Part model, mm, in its own coordinate system. Face numbers are marked on the shaded views. A direction names the side the tool comes from. Coordinates: 2 decimals unless noted, no trailing zeros. Loops run counter-clockwise (first coordinate to the right, second up) from the corner with the lowest first, then second, coordinate; pieces in that order, holes last. Notation, with made-up numbers: (40.25, 45) - (96.25, 45) arc R22 cw to (96.25, 62) - close; hole circle Ø6 at (46.5, 35). An arc over 180 degrees is marked (long way). Use a Markdown table: item, result. Add a question column.
1) Probe probe 1 along Y at (x, z) = (86.5, 50.5); probe 2 along X at (y, z) = (-6.5, 7.5) (3 decimals); probe 3 along Z at (x, y) = (-3, 45.5) (3 decimals). List the from-to ranges inside material, lowest first. Write a range as [from, to].
2) Band-saw the part on B-B (y = 29). Give the cut face in (x, z) (3 decimals), plus the area to 3 significant figures.
3) Drop flat-ended pins along their axis: P1, Ø3, axis at y = 6.5, z = 24, coming from the +X side (3 decimals); P2, Ø6, axis at y = -22.5, z = 30.5, coming from the +X side; P3, Ø16, axis at x = 22.5, z = 40, coming from the +Y side. Give the stop position or say it passes through.
4) Band-saw the part on A-A (x = 87.5). Give the cut face in (y, z) (3 decimals), plus the area to 3 significant figures.
5) Tool access for the marked faces 1, 2, 3 and 4: list every direction of +Z, -Z, +X, -X, +Y, -Y with a clear straight run to the whole face (end or side of a thin tool).
6) Pull direction Y, two halves, no side cores. Call the marked faces 5, 6, 7 and 8: +Y half, -Y half, draft (parallel to the pull), parting line (faces both ways), or undercut.
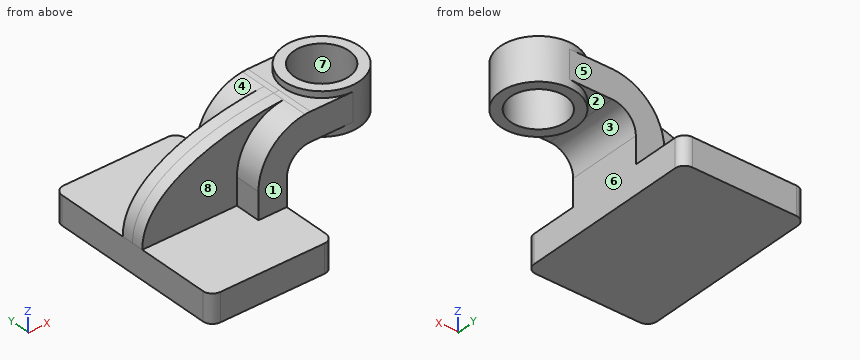
from build123d import *

# Parameters (mm, degrees)
F1_DEPTH = 63.5
F0_W     = 25.4
F0_H     = 19.05
F2_DEPTH = 25.4
F3_DEPTH = 7.9375
F5_R     = 6.35
F6_R     = 18.4889693292
F7_DEPTH = 100.96774064


with BuildPart() as f1:
    # F0 (on Front) → F1 (new body, symmetric)
    with BuildSketch(Plane.XZ):
        Polygon((41.275, -9.525), (41.275, 9.525), (22.225, 9.525), (-41.275, 9.525), (-41.275, -9.525), align=None)
    extrude(amount=F1_DEPTH, both=True)

    # F0 (on Front) → F2 (join, symmetric)
    with BuildSketch(Plane.XZ):
        with BuildLine():
            Line((22.225, 9.525), (41.275, 9.525))
            Line((41.275, 9.525), (41.275, 27.5082))
            ThreePointArc((41.275, 27.5082), (45.9246798487, 38.7335201513), (57.15, 43.3832))
            Line((57.15, 43.3832), (60.325, 43.3832))
            Line((60.325, 43.3832), (60.325, 62.4332))
            Line((60.325, 62.4332), (57.15, 62.4332))
            add(Edge.make_bspline(
                [(53.5324999081, 62.2453460843), (54.7490836223, 62.3182036116), (55.9554653988, 62.3807456949), (57.15, 62.4332)],
                knots=[108.5679461474, 108.5679461474, 108.5679461474, 108.5679461474, 111.7441642872, 111.7441642872, 111.7441642872, 111.7441642872], degree=3))
            ThreePointArc((53.5324999081, 62.2453460843), (31.2068234818, 50.8899710438), (22.225, 27.5082))
            Line((22.225, 27.5082), (22.225, 9.525))
        make_face()
        with Locations((73.025, 52.9082)):
            Rectangle(F0_W, F0_H)
    extrude(amount=F2_DEPTH, both=True)

    # F0 (on Front) → F3 (join, symmetric)
    with BuildSketch(Plane.XZ):
        with BuildLine():
            Line((-41.275, 9.525), (22.225, 9.525))
            Line((22.225, 9.525), (22.225, 27.5082))
            ThreePointArc((22.225, 27.5082), (31.2068234818, 50.8899710438), (53.5324999081, 62.2453460843))
            add(Edge.make_bspline(
                [(-41.275, 9.525), (-41.5565460879, 45.2122684176), (11.9478261389, 59.7549654652), (53.5324999081, 62.2453460843)],
                knots=[0, 0, 0, 0, 108.5679461474, 108.5679461474, 108.5679461474, 108.5679461474], degree=3))
        make_face()
    extrude(amount=F3_DEPTH, both=True)

    # F0 (on Front) → F4 (revolve)
    with BuildSketch(Plane.XZ):
        Polygon((85.725, 62.4332), (85.725, 43.3832), (85.725, 38.1), (111.125, 38.1), (111.125, 66.675), (85.725, 66.675), align=None)
    revolve(axis=Axis((85.725, 0, 52.3875), (0, 0, 1)))

    # F5
    f5_edges = [f1.edges().sort_by_distance(p)[0] for p in [
        (41.275, -63.5, 0),
        (-41.275, -63.5, 0),
        (-41.275, 63.5, 0),
        (41.275, 63.5, 0),
    ]]
    fillet(f5_edges, radius=F5_R)

    # F6 (on face) → F7 (cut)
    with BuildSketch(Plane.XY.offset(66.675)):
        with Locations((85.725, 0)):
            Circle(F6_R)
    extrude(amount=-F7_DEPTH, mode=Mode.SUBTRACT)


solid = f1.part
Answer block:
| question | item | result |
|---|---|---|
| 1 | probe 1 | [-25.39, -18.47], [18.47, 25.39] |
| 1 | probe 2 | [-41.275, 41.275] |
| 1 | probe 3 | [-9.525, 9.525] |
| 2 | outline | (-41.275, -9.525) - (41.275, -9.525) - (41.275, 9.525) - (-41.275, 9.525) - close |
| 2 | area | 1,570 mm2 |
| 3 | P1 | x = 41.275 |
| 3 | P2 | x = 42.45 |
| 3 | P3 | y = 25.4 |
| 4 | outline | (-25.338, 38.1) - (-18.404, 38.1) - (-18.404, 66.675) - (-25.338, 66.675) - close; (18.404, 38.1) - (25.338, 38.1) - (25.338, 66.675) - (18.404, 66.675) - close |
| 4 | area | 396 mm2 |
| 5 | face 1 | +Z, +X, -X, -Y |
| 5 | face 2 | -Z |
| 5 | face 3 | -Z, +Y, -Y |
| 5 | face 4 | +Z, -X, +Y |
| 6 | face 5 | +Y half |
| 6 | face 6 | draft |
| 6 | face 7 | undercut |
| 6 | face 8 | -Y half |
